from build123d import *

# Parameters (mm, degrees)
SKETCH_1_R          = 20
EXTRUDE_1_DEPTH     = 20
SKETCH_2_R          = 15
SKETCH_2_W          = 3
SKETCH_2_H          = 17
CUT_EXTRUDE_1_DEPTH = 35.641016151


with BuildPart() as part:
    # 草图1 → 凸台-拉伸1 (new body)
    with BuildSketch(Plane.XY):
        Circle(SKETCH_1_R)
    extrude(amount=EXTRUDE_1_DEPTH)

    # 草图2 → 切除-拉伸1 (cut, through all)
    with BuildSketch(Plane.XY.offset(20)):
        Circle(SKETCH_2_R)
        with Locations((0, 8.5)):
            Rectangle(SKETCH_2_W, SKETCH_2_H)
    extrude(amount=-CUT_EXTRUDE_1_DEPTH, mode=Mode.SUBTRACT)


solid = part.part
Build history of the part. All positions in model axes, mm. A direction names the side the tool comes from. Give positions to 0.01 mm unless a question says otherwise; leave off trailing zeros. Order: outer loops, then holes, each group sorted by start corner. A loop starts at its lowest first (then second) coordinate and runs counter-clockwise, first axis right, second up. Notation, with made-up numbers: M -14.5,-31.5 L 24.5,-31.5 A17 cw 24.5,-12.5 Z; hole C -30,77 d3. An arc over 180 degrees is marked long. Use one line per item in the form item = value.
Q1. Wall check: probe 1 along Y at (x, z) = (0, 5.5); probe 2 along Y at (x, z) = (4.5, 9.75); probe 3 along X at (y, z) = (-8, 16.75). Give the ranges that are in metal, low to high.
Conclusion:
probe_1 = -20 to -15, 17 to 20
probe_2 = -19.49 to -14.31, 14.31 to 19.49
probe_3 = -18.33 to -12.69, 12.69 to 18.33
Q2. Pull direction Y, two halves, no side cores. Call faces 3 (the flat face through (0, 17, 10)), 4 (the flat face through (1.5, 16, 10)), 5 (the cylindrical face through (-4.336, -19.524, 9.86)), 6 (the flat face through (4, -15, 0)): released by +Y, released by -Y, zero draft, split by the parting line, or undercut.
Conclusion:
face_3 = undercut
face_4 = undercut
face_5 = split by the parting line
face_6 = zero draft
Q3. Slice it at A-A, the plane x = 0. Write the cut outline in (y, z), and give its area (3 significant figures).
Conclusion:
outline = M -20,0 L -15,0 L -15,20 L -20,20 Z; M 17,0 L 20,0 L 20,20 L 17,20 Z
area = 160 mm2
Q4. Slice it at C-C, the plane z = 4.75. Write the cut outline in (x, y).
Conclusion:
outline = C 0,0 d40; hole M -1.5,14.92 A15 ccw long 1.5,14.92 L 1.5,17 L -1.5,17 Z
Q5. Which spindle directions (+Z, -Z, +X, -X, +Y, -Y) get a long thin tool onto all of the face, cutting with end or side? Do faces 1 (the flat face through (-1.5, 16, 10)), 2 (the flat face through (4, -15, 20)). Say none if no direction does.
Conclusion:
face_1 = +Z, -Z
face_2 = +Z, +X, -X, +Y, -Y
Q6. Pin check, flat tips, straight feed: P1, Ø5, axis at x = 7, z = 10.5, coming from the +Y side; P2, Ø2.5, axis at y = 16, z = 6, coming from the +X side; P3, Ø1.5, axis at x = 0, z = 15, coming from the -Y side. Stop position of each tip, or through.
Conclusion:
P1 = 19.49
P2 = 13.51
P3 = -20
Q7. Slice it at B-B, the plane y = 0. Write the cut outline in (x, z), and give its area (3 significant figures).
Conclusion:
outline = M -20,0 L -15,0 L -15,20 L -20,20 Z; M 15,0 L 20,0 L 20,20 L 15,20 Z
area = 200 mm2
